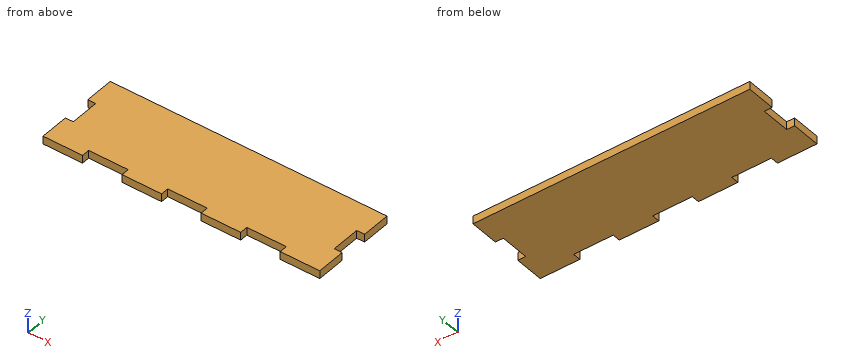
Autodesk Inventor part; units mm, degrees
ref_plane "YZ Plane" through (0, 0, 0) normal (1, 0, 0) x (0, 1, 0)
ref_plane "XZ Plane" through (0, 0, 0) normal (0, 1, 0) x (-1, 0, 0)
ref_plane "XY Plane" through (0, 0, 0) normal (0, 0, 1) x (1, 0, 0)
sketch "Sketch1" plane through (0, 0, 0) normal (0, 0, 1) x (1, 0, 0)
  line L0 (-22.5, 0) -> (-22.5, 3)
  line L1 (-22.5, 3) -> (-37.5, 3)
  line L2 (-37.5, 3) -> (-37.5, 0)
  line L3 (7.5, 0) -> (7.5, 3)
  line L4 (7.5, 3) -> (-7.5, 3)
  line L5 (-7.5, 3) -> (-7.5, 0)
  line L6 (37.5, 0) -> (37.5, 3)
  line L7 (37.5, 3) -> (22.5, 3)
  line L8 (22.5, 3) -> (22.5, 0)
  line L9 (-52.5, 22) -> (-49.5, 22)
  line L10 (-49.5, 22) -> (-49.5, 11)
  line L11 (-49.5, 11) -> (-52.5, 11)
  line L12 (52.5, 11) -> (49.5, 11)
  line L13 (49.5, 11) -> (49.5, 22)
  line L14 (49.5, 22) -> (52.5, 22)
  line L15 (-37.5, 33) -> (-52.5, 33)
  line L16 (52.5, 33) -> (56.4286, 33)
  line L17 (22.5, 33) -> (2.4524, 33)
  line L18 (-7.5, 33) -> (-27.5476, 33)
  line L19 (52.5, 0) -> (52.5, 11)
  line L20 (52.5, 22) -> (52.5, 33)
  line L21 (37.5, 0) -> (52.5, 0)
  line L22 (7.5, 0) -> (22.5, 0)
  line L23 (-52.5, 0) -> (-37.5, 0)
  line L24 (-22.5, 0) -> (-7.5, 0)
  line L25 (-52.5, 33) -> (-52.5, 22)
  line L26 (-52.5, 11) -> (-52.5, 0)
  line L27 (-37.5, 33) -> (57.8569, 33)
  point P0 (0, 0)
  point P1 (0, 30)
  dimension "d46" = 105
  dimension "d48" = 33
  dimension "d49" = 52.5
  dimension "d50" = 0
  dimension "d53" = 0
  dimension "d58" = 11
  dimension "d59" = 11
  dimension "d61" = 15
  dimension "d62" = 7.5
  dimension "d63" = 3
  dimension "d64" = 3
  dimension "d65" = 3
extrude "Extrusion1" add sketch "Sketch1" along normal blind 3
equation "\"d46\" = shelfWs"
equation "\"d48\" = shelfD"
equation "\"d58\" = 0.333333 * shelfD - tol"
equation "\"d59\" = 0.333333 * shelfD + 2 * tol"
equation "\"d24\" = tt"
equation "\"d0\" = 0.5 * shelfWs"
equation "\"tt\" = 3"
equation "\"tol\" = 0"
equation "\"d2\" = shelfD"
equation "\"d4\" = tt"
equation "\"tiroir\" = 1"
equation "\"nHoles\" = 4"
equation "\"shelfH\" = 35"
equation "\"shelfWs\" = 105"
equation "\"d47\" = 0.5 * shelfWs"
properties part number "back"
Can you work these out from the model? Positions are in its coordinate system, mm. Give positions to 0.01 mm unless a question says otherwise; leave off trailing zeros. Order: outer loops, then holes, each group sorted by start corner. A loop starts at its lowest first (then second) coordinate and runs counter-clockwise, first axis right, second up. Notation, with made-up numbers: M 74,30 L 109,30 A7 cw 109,43 Z; hole C 47.5,78 d5. An arc over 180 degrees is marked long. Write item = value, one per line. Start each with the question number.
Q1. Will these pins go through, and if not, where does the flat tip stop? pin 1 Ø0.9 at (y, z) = (15, 2) entering from +X; pin 2 Ø1 at (x, z) = (-36, 0.5) entering from -Y.
Q2. Suppose I cut it at B-B (y = 19). Write out the boundary of the cut face in (x, z), plus the area to 3 significant figures.
Q3. I need wall thicknesses on probe 1 along Y at (x, z) = (-25.5, 1.45); probe 2 along X at (y, z) = (16, 0.4). Which ranges of each line are inside material? Lowest first, please. Write a range as [from, to].
Q4. Suppose I cut it at A-A (z = 0.95). Write out the boundary of the cut face in (x, y), plus the area to 3 significant figures.
Q5. Suppose I cut it at C-C (x = -32). Write out the boundary of the cut face in (y, z).
Check result:
q1.pin_1 = 49.5
q1.pin_2 = 3
q2.outline = M -49.5,0 L 49.5,0 L 49.5,3 L -49.5,3 Z
q2.area = 297 mm2
q3.probe_1 = [3, 33]
q3.probe_2 = [-49.5, 49.5]
q4.outline = M -52.5,0 L -37.5,0 L -37.5,3 L -22.5,3 L -22.5,0 L -7.5,0 L -7.5,3 L 7.5,3 L 7.5,0 L 22.5,0 L 22.5,3 L 37.5,3 L 37.5,0 L 52.5,0 L 52.5,11 L 49.5,11 L 49.5,22 L 52.5,22 L 52.5,33 L -52.5,33 L -52.5,22 L -49.5,22 L -49.5,11 L -52.5,11 Z
q4.area = 3,260 mm2
q5.outline = M 3,0 L 33,0 L 33,3 L 3,3 Z
